Can you work these out from the model? Positions are in its coordinate system, mm. A direction names the side the tool comes from. Round coordinates to 2 decimals unless told otherwise and drop trailing zeros. Write each loop counter-clockwise with the first axis right and the second up, starting at its lowest first coordinate (ties: lowest second). Pieces come first, ordered by that corner, then holes.
Q1. We'd pull the mould along X, two halves only. Please class faces 3 (the flat face through (-24.695, 14.257, 36.031)), 4 (the flat face through (-52.5, 16, 35)), 5 (the flat face through (1, -1.6, 35)): +X half, -X half, draft (parallel to the pull), parting line (faces both ways), or undercut.
Q2. I'm going to push flat-ended pins straight in: pin 1 Ø1 at (x, z) = (-4, 52) entering from +Y; pin 2 Ø1.5 at (x, z) = (14.5, 59.5) entering from +Y; pin 3 Ø1 at (x, y) = (-18, 28) entering from +Z; pin 4 Ø3 at (x, y) = (-15.5, 26) entering from -Z. Where does each tip first touch, or does it pass through?
Q3. If we section it at B-B (z = 33): Please give me the cut outline in (x, y).
Q4. If we section it at C-C (x = -36.5): Please give me the cut outline in (y, z), plus the area to 3 significant figures.
Q5. Please list where these lines run through material, in increasing order: line 1 along Z through (x, y) = (-29.5, 23.5); line 2 along X through (y, z) = (8, 15); line 3 along X through (y, z) = (24, 41).
Q6. For faces 1 (the cylindrical face through (-0.11, 2.32, 36.03)), 2 (the flat face through (-1, 1, 70)), which set-ups out of +Z, -Z, +X, -X, +Y, -Y let a thin tool reach every point of the face, with its end or its side?
Q7. If we section it at D-D (y = 17): Please give me the cut outline in (x, z).
Q8. If we section it at A-A (y = 7.5): Please give me the cut outline in (x, z), plus the area to 3 significant figures.
from build123d import *

# Parameters (mm, degrees)
BOSS_EXTRU_1_DEPTH = 70
CONG_1_R           = 15
ESQUISSE2_W        = 105
ESQUISSE2_H        = 35
BOSS_EXTRU_2_DEPTH = 3


with BuildPart() as part:
    # Esquisse1 → Boss.-Extru.1 (new body)
    with BuildSketch(Plane.XY):
        Polygon((0, 0), (48.5, 28.001488056), (48.5, 33.4), (52.5, 33.4), (52.5, -1.6), (-52.5, -1.6), (-52.5, 33.4), (-48.5, 33.4), (-48.5, 28.001488056), align=None)
    extrude(amount=BOSS_EXTRU_1_DEPTH)

    # Congé1
    # the kernel refuses this fillet: 15 mm, written as the material it adds along each edge
    with BuildSketch(Plane(origin=(0, 0, 0), x_dir=(0.866025403784438, 0.5000000000000011, 0), z_dir=(0, 0, 1))) as cong_1_piece_1:
        with BuildLine():
            CenterArc((CONG_1_R * 0.57735026919, CONG_1_R), CONG_1_R, 210, 60)
            Line((-CONG_1_R * 0.288675134595, CONG_1_R * 0.5), (-CONG_1_R * 0.305995642671, CONG_1_R * 0.49))
            Line((-CONG_1_R * 0.305995642671, CONG_1_R * 0.49), (-CONG_1_R * 0.0115470053838, -CONG_1_R * 0.02))
            Line((-CONG_1_R * 0.0115470053838, -CONG_1_R * 0.02), (CONG_1_R * 0.57735026919, -CONG_1_R * 0.02))
            Line((CONG_1_R * 0.57735026919, -CONG_1_R * 0.02), (CONG_1_R * 0.57735026919, 0))
        make_face()
    extrude(amount=70)
    with BuildSketch(Plane(origin=(48.5, 28.001488056, 0), x_dir=(-0.8660254037844379, -0.5000000000000011, 0), z_dir=(0, 0, 1))) as cong_1_piece_2:
        with BuildLine():
            CenterArc((8.181897743, -15), CONG_1_R, 90, 46.502986309)
            Line((-2.699255972, -4.675248486), (-2.916879046, -4.468753456))
            ThreePointArc((-2.916879046, -4.468753456), (-1.609435607, -2.187624243), (-0.259807621, 0.15))
            Line((-0.259807621, 0.15), (0, 0.3))
            Line((0, 0.3), (8.181897743, 0.3))
            Line((8.181897743, 0.3), (8.181897743, 0))
        make_face()
    extrude(amount=70)
    with BuildSketch(Plane(origin=(-48.5, 28.001488056, 0), x_dir=(0, 1, 0), z_dir=(0, 0, 1))) as cong_1_piece_3:
        with BuildLine():
            CenterArc((8.899432185, -14.585731297), CONG_1_R, 103.497013691, 46.502986309)
            Line((-4.090948872, -7.085731297), (-4.350756493, -6.935731297))
            Line((-4.350756493, -6.935731297), (-0.259807621, 0.15))
            Line((-0.259807621, 0.15), (0, 0.3))
            ThreePointArc((0, 0.3), (2.699255972, 0.3), (5.328493539, 0.291714626))
            Line((5.328493539, 0.291714626), (5.398511944, 0))
        make_face()
    extrude(amount=70)

    # Esquisse2 → Boss.-Extru.2 (add)
    with BuildSketch(Plane.XY):
        with Locations((0, 15.9)):
            Rectangle(ESQUISSE2_W, ESQUISSE2_H)
    extrude(amount=BOSS_EXTRU_2_DEPTH)


solid = part.part
A:
1. face 3: undercut
1. face 4: -X half
1. face 5: draft
2. pin 1: stops at y = 3.01
2. pin 2: stops at y = 8.8
2. pin 3: stops at z = 3
2. pin 4: stops at z = 0
3. outline: (-52.5, -1.6) - (52.5, -1.6) - (52.5, 33.4) - (48.5, 33.4) arc R15 cw to (41.41, 23.91) - (7.5, 4.33) arc R15 cw to (-7.5, 4.33) - (-41.41, 23.91) arc R15 cw to (-48.5, 33.4) - (-52.5, 33.4) - close
4. outline: (-1.6, 0) - (33.4, 0) - (33.4, 3) - (21.07, 3) - (21.07, 70) - (-1.6, 70) - close
4. area: 1,620 mm2
5. line 1: z = 0 to 3
5. line 2: x = -52.5 to -13.86, 13.86 to 52.5
5. line 3: x = -52.5 to -41.57, 41.57 to 52.5
6. face 1: +Z, +Y
6. face 2: +Z, +X, -X, +Y, -Y
7. outline: (-52.5, 0) - (52.5, 0) - (52.5, 70) - (29.44, 70) - (29.44, 3) - (-29.44, 3) - (-29.44, 70) - (-52.5, 70) - close
8. outline: (-52.5, 0) - (52.5, 0) - (52.5, 70) - (12.99, 70) - (12.99, 3) - (-12.99, 3) - (-12.99, 70) - (-52.5, 70) - close
8. area: 5,610 mm2
